Autodesk Inventor part; units mm, degrees
ref_plane "YZ Plane" through (0, 0, 0) normal (1, 0, 0) x (0, 1, 0)
ref_plane "XZ Plane" through (0, 0, 0) normal (0, 1, 0) x (-1, 0, 0)
ref_plane "XY Plane" through (0, 0, 0) normal (0, 0, 1) x (1, 0, 0)
sketch "main" plane through (0, 0, 0) normal (0, 0, 1) x (1, 0, 0)
  circle A0 centre (-38.8868, 18.5788) radius 2.2479
  circle A1 centre (2.3882, 18.5788) radius 2.2479
  circle A2 centre (2.3882, 43.9788) radius 2.1844
  arc A3 (3.9757, 48.4689) -> (3.4489, 48.6217) centre (2.3882, 43.9788) ccw
  arc A4 (3.9552, 14.0814) -> (7.1507, 18.5788) centre (2.3882, 18.5788) ccw
  circle A5 centre (-38.8868, 31.2788) radius 2.0955
  circle A6 centre (-38.8868, 5.8788) radius 2.0955
  arc A7 (-44.9109, 33.2868) -> (-45.2368, 31.2788) centre (-38.8868, 31.2788) ccw
  arc A8 (-45.2368, 5.8788) -> (-36.7975, -0.1177) centre (-38.8868, 5.8788) ccw
  circle A9 centre (-32.5368, 50.3288) radius 2.0955
  arc A10 (-31.1226, 56.5193) -> (-38.5609, 52.3368) centre (-32.5368, 50.3288) ccw
  line L0 (-44.9109, 33.2868) -> (-38.5609, 52.3368)
  line L1 (3.4489, 48.6217) -> (-31.1226, 56.5193)
  line L2 (3.9552, 14.0814) -> (-36.7975, -0.1177)
  line L3 (-45.2368, 31.2788) -> (-45.2368, 5.8788)
  arc A11 (7.1507, 43.9788) -> (3.4489, 48.6217) centre (2.3882, 43.9788) ccw
  line L4 (7.1507, 43.9788) -> (7.1507, 18.5788)
  circle A12 centre (2.3882, 31.2788) radius 2.1844
  point P0 (-4.3882, 4.0845)
  dimension "d11" = 4.4958
  dimension "d12" = 4.4958
  dimension "d13" = 9.525
  dimension "d14" = 9.525
  dimension "d15" = 4.191
  dimension "d16" = 4.191
  dimension "d17" = 41.275
  dimension "d18" = 41.275
  dimension "d19" = 25.4
  dimension "d20" = 4.3688
  dimension "d21" = 12.7
sketch "Sketch1" plane through (0, 0, 0) normal (0, 0, 1) x (1, 0, 0)
  circle A0 centre (-12.7, 0) radius 2.2479
  circle A1 centre (-12.7, 41.275) radius 2.2479
  circle A2 centre (-38.1, 41.275) radius 2.1844
  arc A3 (-42.5901, 42.8625) -> (-42.7429, 42.3356) centre (-38.1, 41.275) ccw
  arc A4 (-8.2027, 42.842) -> (-12.7, 46.0375) centre (-12.7, 41.275) ccw
  circle A5 centre (-25.4, 0) radius 2.0955
  circle A6 centre (0, 0) radius 2.0955
  arc A7 (-27.408, -6.0241) -> (-25.4, -6.35) centre (-25.4, 0) ccw
  arc A8 (0, -6.35) -> (5.9964, 2.0893) centre (0, 0) ccw
  circle A9 centre (-44.45, 6.35) radius 2.0955
  arc A10 (-50.6405, 7.7642) -> (-46.458, 0.3259) centre (-44.45, 6.35) ccw
  line L0 (-27.408, -6.0241) -> (-46.458, 0.3259)
  line L1 (-42.7429, 42.3356) -> (-50.6405, 7.7642)
  line L2 (-8.2027, 42.842) -> (5.9964, 2.0893)
  line L3 (-25.4, -6.35) -> (0, -6.35)
  arc A11 (-38.1, 46.0375) -> (-42.7429, 42.3356) centre (-38.1, 41.275) ccw
  line L4 (-38.1, 46.0375) -> (-12.7, 46.0375)
  circle A12 centre (-25.4, 41.275) radius 2.1844
  point P0 (0, 0)
  point P1 (-42.5901, 42.8625)
extrude "Extrusion1" add sketch "Sketch1" along normal blind 1.5875
properties part number "gusset" material "Acetal Resin, White"
Source: CAD feature listing. Evaluate the final solid. Frame: model axes, mm. Round coordinates to 2 decimals unless told otherwise and drop trailing zeros. Write each loop counter-clockwise with the first axis right and the second up, starting at its lowest first coordinate (ties: lowest second). Pieces come first, ordered by that corner, then holes. Notation, with made-up numbers: M 14,47 L 73,47 A22 cw 73,69 Z; hole C -14,-20.5 d11. An arc over 180 degrees is marked long. Use CSV: the item, a comma, the result in double quotes. Start each with the question number.
Q1. First-contact query: P1, Ø7, axis at x = -25.4, y = 41.275, coming from the -Z side. Flat tip, straight axial feed; report the tip coordinate or a pass-through.
Q2. Line query: line 1 (Y direction, x = -25.4, z = 1.15); line 2 (Y direction, x = -12.7, z = 0.3); line 3 (X direction, y = 41.5, z = 1.45). Output: solid intervals per line, ascending. Write a range as from..to.
Q3. Cut plane C-C on z = 1.1. Count the separate pieces of the cut face and the enclosed holes in it, plus the area to 3 significant figures.
Q4. Cut plane A-A on x = -44.45. Output: boundary loops of the cut face in (y, z), plus the area to 3 significant figures.
Q5. Pull-direction query (X, two-part tool) for faces 1 (the face through (-24.23, 39.43, 0.78)), 2 (the face through (-26, 46.038, 1)), 3 (the face through (5.225, -3.609, 0.783)); classes: +X half, -X half, draft (parallel to the pull), parting line (faces both ways), or undercut.
Q6. Cut plane B-B on y = 6.35. Output: boundary loops of the cut face in (x, z).
Q7. Cut plane D-D on y = 17.5. Output: boundary loops of the cut face in (x, z).
Results found:
1,P1,"z = 0"
2,line 1,"-6.35..-2.1, 2.1..39.09, 43.46..46.04"
2,line 2,"-6.35..-2.25, 2.25..39.03, 43.52..46.04"
2,line 3,"-42.93..-40.27, -35.93..-27.57, -23.23..-14.94, -10.46..-7.74"
3,separate pieces,"1"
3,enclosed holes,"7"
3,area,"2,250 mm^2"
4,outline,"M -0.34,0 L 4.25,0 L 4.25,1.59 L -0.34,1.59 Z; M 8.45,0 L 34.86,0 L 34.86,1.59 L 8.45,1.59 Z"
4,area,"49.2 mm^2"
5,face 1,"undercut"
5,face 2,"draft"
5,face 3,"+X half"
6,outline,"M -50.8,0 L -46.55,0 L -46.55,1.59 L -50.8,1.59 Z; M -42.35,0 L 4.51,0 L 4.51,1.59 L -42.35,1.59 Z"
7,outline,"M -48.42,0 L 0.63,0 L 0.63,1.59 L -48.42,1.59 Z"
